The model under review builds one solid part; all positions refer to its coordinate system, in mm. A direction names the side the tool comes from. Coordinates: 2 decimals unless noted, no trailing zeros. Loops run counter-clockwise (first coordinate to the right, second up) from the corner with the lowest first, then second, coordinate; pieces in that order, holes last. Notation, with made-up numbers: (-37.5, 76) - (-0.5, 76) arc R17 ccw to (-0.5, 82) - close; hole circle Ø10 at (85.5, 44.25). An arc over 180 degrees is marked (long way). One line per item, written item: value. Start each with the question number.
1. To check wall thickness, follow line 1 (Y direction, x = -15.5, z = 40); line 2 (Z direction, x = -0.5, y = -15); line 3 (Z direction, x = 5, y = 0). State the ranges of each line that lie inside material, in increasing order.
2. We need section A-A, the plane z = 44. Give the boundary of the cut face in (x, y), then the cut area to 3 significant figures.
3. We need section C-C, the plane x = -15.5. Give the boundary of the cut face in (y, z), then the cut area to 3 significant figures.
4. We need section B-B, the plane y = 0. Give the boundary of the cut face in (x, z), then the cut area to 3 significant figures.
5. Insertion check: P1, Ø5, axis at x = 15.5, y = 15.5, coming from the -Z side; P2, Ø2, axis at x = -14.5, y = 16, coming from the +Z side; P3, Ø1.2, axis at x = 15.5, y = 15, coming from the +Z side; P4, Ø6, axis at x = 12.5, y = 0.5, coming from the +Z side. Each pin has a flat end and moves straight along its axis. Give the tip position at first contact, or say it passes through.
6. For faces 4 (the face through (15.24, 17.483, 42.07)), 5 (the face through (0, -21.15, 23)), list the 3-axis set-ups (+Z, -Z, +X, -X, +Y, -Y) from which the entire face can be reached by the end or side of a thin tool; tool diameter is ignored.
7. Mouldability with a two-part tool opening along X and no side actions: class faces 1 (the face through (0, 21.15, 23)), 2 (the face through (-0.54, 2.44, 59.35)), 3 (the face through (-15.76, 17.483, 42.07)) as +X half, -X half, draft (parallel to the pull), parting line (faces both ways), or undercut.
8. We need section D-D, the plane z = 53. Give the boundary of the cut face in (x, y).
Solid Edge part; units mm, degrees
sketch "Sketch1" plane through (0, 0, 0) normal (0, 0, 1) x (1, 0, 0)
  line L0 (-21.2, -21.15) -> (21.2, -21.15)
  line L1 (21.2, -21.15) -> (21.2, 21.15)
  line L2 (21.2, 21.15) -> (-21.2, 21.15)
  line L3 (-21.2, 21.15) -> (-21.2, -21.15)
extrude "Protrusion1" add sketch "Sketch1" along normal blind 47
chamfer "Chamfer_1" distance 3 angle 45 4 edges at (21.2, -21.15, 23.5) (-21.2, -21.15, 23.5) (-21.2, 21.15, 23.5) (21.2, 21.15, 23.5)
sketch "Sketch2" plane through (0, 0, 47) normal (0, 0, 1) x (1, 0, 0)
  circle A0 centre (0, 0) radius 2.5
extrude "ExtrudedProtrusion_2" add sketch "Sketch2" along normal blind 23.5
sketch "Sketch3" plane through (0, 0, 47) normal (0, 0, 1) x (1, 0, 0)
  circle A0 centre (-15.5, 15.5) radius 2
  circle A1 centre (-15.5, -15.5) radius 2
  circle A2 centre (15.5, -15.5) radius 2
  circle A3 centre (15.5, 15.5) radius 2
extrude "ExtrudedCutout_1" cut sketch "Sketch3" against normal blind 10
sketch "Sketch4" plane through (0, 0, 47) normal (0, 0, 1) x (1, 0, 0)
  circle A0 centre (0, 0) radius 11
extrude "ExtrudedProtrusion_3" add sketch "Sketch4" along normal blind 1.5
Findings below:
1. line 1: -21.15 to -17.5, -13.5 to 13.5, 17.5 to 21.15
1. line 2: 0 to 47
1. line 3: 0 to 48.5
2. outline: (-21.2, -18.15) - (-18.2, -21.15) - (18.2, -21.15) - (21.2, -18.15) - (21.2, 18.15) - (18.2, 21.15) - (-18.2, 21.15) - (-21.2, 18.15) - close; hole circle Ø4 at (-15.5, -15.5); hole circle Ø4 at (-15.5, 15.5); hole circle Ø4 at (15.5, -15.5); hole circle Ø4 at (15.5, 15.5)
2. area: 1,730 mm2
3. outline: (-21.15, 0) - (21.15, 0) - (21.15, 47) - (17.5, 47) - (17.5, 37) - (13.5, 37) - (13.5, 47) - (-13.5, 47) - (-13.5, 37) - (-17.5, 37) - (-17.5, 47) - (-21.15, 47) - close
3. area: 1,910 mm2
4. outline: (-21.2, 0) - (21.2, 0) - (21.2, 47) - (11, 47) - (11, 48.5) - (2.5, 48.5) - (2.5, 70.5) - (-2.5, 70.5) - (-2.5, 48.5) - (-11, 48.5) - (-11, 47) - (-21.2, 47) - close
4. area: 2,140 mm2
5. P1: z = 0
5. P2: z = 47
5. P3: z = 37
5. P4: z = 48.5
6. face 4: +Z
6. face 5: +Z, -Z, +X, -X, -Y
7. face 1: draft
7. face 2: parting line
7. face 3: undercut
8. outline: circle Ø5 at (0, 0)
